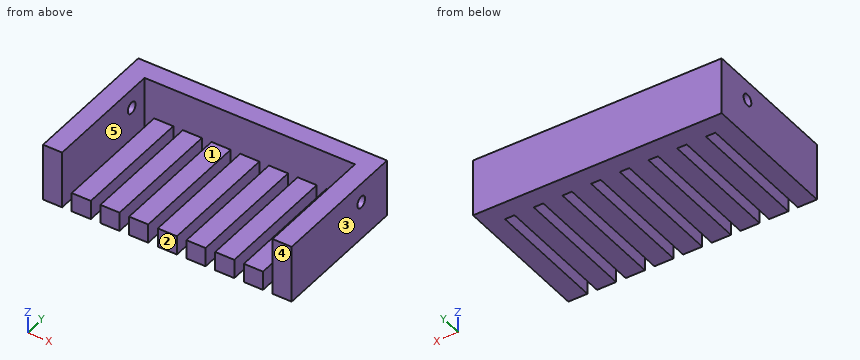
```python
from build123d import *

# Parameters (mm, degrees)
PAD_DEPTH         = 10
PAD001_DEPTH      = 20
SKETCH002_R       = 3
POCKET_DEPTH      = 10.001
POCKET_DEPTH_BACK = -120.001


with BuildPart() as part:
    # Sketch → Pad (new body)
    with BuildSketch(Plane.XY):
        Polygon((-65, 0), (-55, 0), (-55, 64), (-50, 64), (-50, 0), (-40, 0), (-40, 64), (-35, 64), (-35, 0), (-25, 0), (-25, 64), (-20, 64), (-20, 0), (-10, 0), (-10, 64), (-5, 64), (-5, 0), (5, 0), (5, 64), (10, 64), (10, 0), (20, 0), (20, 64), (25, 64), (25, 0), (35, 0), (35, 64), (40, 64), (40, 0), (50, 0), (50, 64), (55, 64), (55, 0), (65, 0), (65, 74), (-65, 74), align=None)
    extrude(amount=PAD_DEPTH)

    # Sketch001 (on Face38 of Pad) → Pad001 (join)
    with BuildSketch(Plane.XY.offset(10)):
        Polygon((-55, 0), (-65, 0), (-65, 74), (65, 74), (65, 0), (55, 0), (55, 64), (-55, 64), align=None)
    extrude(amount=PAD001_DEPTH)

    # Sketch002 (on Face34 of Pad001) → Pocket (cut, two sides)
    with BuildSketch(Plane.YZ.offset(-55)) as pocket_sk:
        with Locations((54, 20)):
            Circle(SKETCH002_R)
    extrude(amount=-POCKET_DEPTH, mode=Mode.SUBTRACT)
    extrude(pocket_sk.sketch, amount=-POCKET_DEPTH_BACK, mode=Mode.SUBTRACT)


solid = part.part
```
Input: part model. Units: mm. Frame: model coordinates. Face numbers are marked on the shaded views. A direction names the side the tool comes from. Give positions to 0.01 mm unless a question says otherwise; leave off trailing zeros. Order: outer loops, then holes, each group sorted by start corner. A loop starts at its lowest first (then second) coordinate and runs counter-clockwise, first axis right, second up. Notation, with made-up numbers: (-15.75, 45) - (40.25, 45) arc R21 ccw to (40.25, 74) - close; hole circle Ø1 at (-24.5, 40). An arc over 180 degrees is marked (long way). Put each result on its own line as item: value.
Item 1: Section query A-A, the plane z = 20. Return loops of the section in (x, y), then the cut area to 3 significant figures.
Found:
outline: (-65, 0) - (-55, 0) - (-55, 51) - (-65, 51) - close; (-65, 57) - (-55, 57) - (-55, 64) - (55, 64) - (55, 57) - (65, 57) - (65, 74) - (-65, 74) - close; (55, 0) - (65, 0) - (65, 51) - (55, 51) - close
area: 2,460 mm^2
Item 2: Section query B-B, the plane x = -18. Return loops of the section in (y, z).
Found:
outline: (0, 0) - (74, 0) - (74, 30) - (64, 30) - (64, 10) - (0, 10) - close
Item 3: Access query for the marked faces 1 and 2. Directions: +Z, -Z, +X, -X, +Y, -Y. A direction counts if a zero-diameter tool reaches every point of the face in a straight line with its end or side. Return the directions, or none.
Found:
face 1: +Z, -Y
face 2: +Z, -Z, +X, -X, -Y
Item 4: Contact query for flat-ended pins moving along their axis: pin 1 (4 mm diameter, centred on x = -40, z = 4.5, fed in from -Y); pin 2 (5 mm diameter, centred on x = -19.5, z = 17.5, fed in from -Y); pin 3 (3 mm diameter, centred on x = -44, y = 47, fed in from +Z). Output: stop coordinate, or through.
Found:
pin 1: stops at y = 0
pin 2: stops at y = 64
pin 3: stops at z = 10
Item 5: Ray query, L1, parallel to X at y = 27, z = 18.5; L2, parallel to Z at x = -59, y = 54; L3, parallel to Y at x = 61.75, z = 20. Return the intervals inside material, ascending. Write a range as from..to.
Found:
L1: x = -65..-55, 55..65
L2: z = 0..17, 23..30
L3: y = 0..51, 57..74
Item 6: Draft query along X for the marked faces 3, 4 and 5. Return one class per face: +X half, -X half, draft (parallel to the pull), parting line (faces both ways), or undercut.
Found:
face 3: +X half
face 4: draft
face 5: undercut
Item 7: Section query C-C, the plane y = 54. Count the separate pieces of the cut face and the enclosed holes in it, then the cut area to 3 significant figures.
Found:
separate pieces: 11
enclosed holes: 0
area: 1,180 mm^2
